Autodesk Fusion 360 part; units mm, degrees
sketch "Base" plane through (0, 0, 0) normal (0, 1, 0) x (1, 0, 0)
  circle A0 centre (0, 0) radius 7
  dimension "d1" = 14
extrude "Extrude1" add sketch "Base" along normal blind 4
sketch "Pin" plane through (0, 4, 0) normal (0, 1, 0) x (-1, 0, 0)
  circle A0 centre (0, 0) radius 7
  circle A1 centre (0, 0) radius 2.875
  dimension "d4" = 5.75
extrude "Extrude2" add sketch "Pin" along normal blind 25 contours A1
hole "Hole1" at (-0.0382, 0, -0.0078) direction (0, 1, 0) diameter 2 end through all
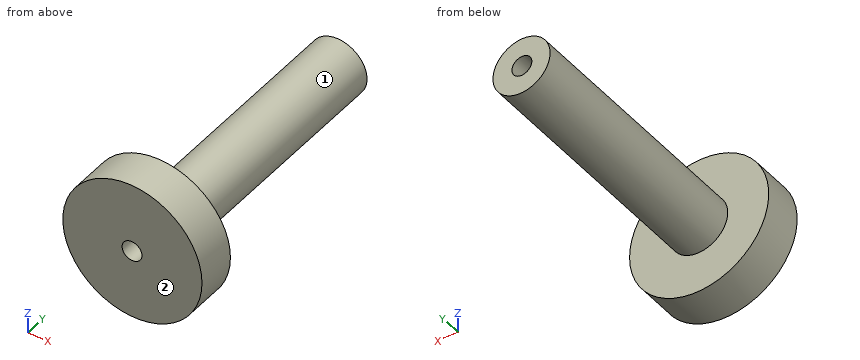
CAD build for the part. Positions are in the model's coordinates, mm. Face numbers are marked on the shaded views. A direction names the side the tool comes from. Round coordinates to 2 decimals unless told otherwise and drop trailing zeros. Order: outer loops, then holes, each group sorted by start corner. A loop starts at its lowest first (then second) coordinate and runs counter-clockwise, first axis right, second up. Notation, with made-up numbers: (-17.75, 43) - (18.25, 43) arc R9 cw to (18.25, 52) - close; hole circle Ø10 at (-5, 40). An arc over 180 degrees is marked (long way). Answer as CSV lines item,"result". Start each with the question number.
1. Saw through at A-A, the plane z = 0. Write the cut outline in (x, y) (3 decimals).
2. Drill centre lines: L1, parallel to Y at x = 0, z = -5.75; L2, parallel to X at y = 7, z = -0.25; L3, parallel to Z at x = 1.75, y = 7.75. Where is each one in solid material? Low to high. Write a range as [from, to].
3. Saw through at C-C, the plane x = -6. Write the cut outline in (y, z), and give its area (3 significant figures).
4. Saw through at D-D, the plane z = -3.5. Write the cut outline in (x, y), and give its area (3 significant figures).
5. Saw through at B-B, the plane y = 3.5. Write the cut outline in (x, z), and give its area (3 significant figures).
6. Pin check, flat tips, straight feed: pin 1 (5 mm diameter, centred on x = -3.5, z = 4, fed in from +Y); pin 2 (5 mm diameter, centred on y = 13.5, z = -3, fed in from +X); pin 3 (1.8 mm diameter, centred on x = -0.04, z = -0.01, fed in from +Y); pin 4 (3 mm diameter, centred on y = 9, z = 3.5, fed in from -X). Stop position of each tip, or through.
7. Tool access for the marked faces 1 and 2: list every direction of +Z, -Z, +X, -X, +Y, -Y with a clear straight run to the whole face (end or side of a thin tool).
Model answer:
1,outline,"(-7, 0) - (-1.038, 0) - (-1.038, 29) - (-2.875, 29) - (-2.875, 4) - (-7, 4) - close; (0.962, 0) - (7, 0) - (7, 4) - (2.875, 4) - (2.875, 29) - (0.962, 29) - close"
2,L1,"y = [0, 4]"
2,L2,"x = [-2.86, -1.01], [0.93, 2.86]"
2,L3,"z = [-2.28, 2.28]"
3,outline,"(0, -3.61) - (4, -3.61) - (4, 3.61) - (0, 3.61) - close"
3,area,"28.8 mm²"
4,outline,"(-6.06, 0) - (6.06, 0) - (6.06, 4) - (-6.06, 4) - close"
4,area,"48.5 mm²"
5,outline,"circle Ø14 at (0, 0); hole circle Ø2 at (-0.04, -0.01)"
5,area,"151 mm²"
6,pin 1,"stops at y = 29"
6,pin 2,"stops at x = 2.83"
6,pin 3,"passes through"
6,pin 4,"stops at x = -2.07"
7,face 1,"+Y"
7,face 2,"+Z, -Z, +X, -X, -Y"
